from build123d import *

# Parameters (mm, degrees)
F0_W     = 68.58
F0_H     = 53.34
F0_R     = 1.5875
F1_DEPTH = 3.175


with BuildPart() as f1:
    # F0 (on Top) → F1 (new body)
    with BuildSketch(Plane.XY):
        with Locations((34.29, -26.67)):
            Rectangle(F0_W, F0_H)
        with Locations((13.97, -50.8)):
            Circle(F0_R, mode=Mode.SUBTRACT)
        with BuildLine():
            ThreePointArc((67.6275, -45.72), (64.9174679849, -46.8425320151), (66.04, -44.1325))
            ThreePointArc((66.04, -44.1325), (67.1625320151, -44.5974679849), (67.6275, -45.72))
        make_face(mode=Mode.SUBTRACT)
        with Locations((15.24, -2.54)):
            Circle(F0_R, mode=Mode.SUBTRACT)
        with BuildLine():
            ThreePointArc((67.6275, -17.78), (67.1625320151, -18.9025320151), (66.04, -19.3675))
            ThreePointArc((66.04, -19.3675), (64.9174679849, -16.6574679849), (67.6275, -17.78))
        make_face(mode=Mode.SUBTRACT)
    extrude(amount=F1_DEPTH)


solid = f1.part
Design review of the part built by this model. Coordinates are the model's own, in mm. Coordinates: 2 decimals unless noted, no trailing zeros. Order: outer loops, then holes, each group sorted by start corner. A loop starts at its lowest first (then second) coordinate and runs counter-clockwise, first axis right, second up.
Item 1: Take a section at A-A, the plane y = -50.8. Write out the cut boundary in (x, z) (1 decimal), then the cut area to 3 significant figures.
Item 2: The part is to be moulded in two halves that separate along X. For faces 1 (the cylindrical face through (16.754, -2.063, 1.565)), 2 (the flat face through (68.58, -27, 2)), 3 (the flat face through (34, -53.34, 2)), 4 (the flat face through (0, -27, 2)), say which applies: pulls with the +X half, pulls with the -X half, needs draft (parallel to the pull), parting line crosses it, or undercut.
Item 3: For line 1 (Y direction, x = 66.04, z = 1.3); line 2 (X direction, y = -45.72, z = 1.65); line 3 (Y direction, x = 13.97, z = 1.95), list the stretches that pass through material, from the lowest coordinate up.
Item 4: For pin 1 Ø2.5 at (x, y) = (66.04, -45.72) entering from -Z; pin 2 Ø1 at (x, z) = (31.5, 0.5) entering from +Y, all flat-tipped, find the tip position at first contact; note any pin that passes through.
The answers:
1. outline: (0, 0) - (12.4, 0) - (12.4, 3.2) - (0, 3.2) - close; (15.6, 0) - (68.6, 0) - (68.6, 3.2) - (15.6, 3.2) - close
1. area: 208 mm2
2. face 1: undercut
2. face 2: pulls with the +X half
2. face 3: needs draft
2. face 4: pulls with the -X half
3. line 1: y = -53.34 to -47.31, -44.13 to -19.37, -16.19 to 0
3. line 2: x = 0 to 64.45, 67.63 to 68.58
3. line 3: y = -53.34 to -52.39, -49.21 to -3.49, -1.59 to 0
4. pin 1: passes through
4. pin 2: stops at y = 0
